Source: CAD feature listing. Evaluate the final solid. Frame: model axes, mm. Round coordinates to 2 decimals unless told otherwise and drop trailing zeros. Write each loop counter-clockwise with the first axis right and the second up, starting at its lowest first coordinate (ties: lowest second). Pieces come first, ordered by that corner, then holes. Notation, with made-up numbers: M 10.5,21.5 L 32.5,21.5 A20 cw 32.5,38.5 Z; hole C 13.25,-19.75 d1. An arc over 180 degrees is marked long. Answer in a Markdown table with one row per item. Add a question column.
Item 1: Cut plane B-B on x = 4.5. Return loops of the section in (y, z), and give its area (3 significant figures).
Item 2: Cut plane A-A on x = -20. Return loops of the section in (y, z).
Item 3: Contact query for flat-ended pins moving along their axis: pin 1 (1.5 mm diameter, centred on x = 76.5, z = 1, fed in from -Y); pin 2 (0.9 mm diameter, centred on x = -11, z = 1, fed in from +Y); pin 3 (0.9 mm diameter, centred on y = 53, z = 1, fed in from +X). Output: stop coordinate, or through.
Item 4: Cut plane C-C on y = -30. Return loops of the section in (x, z).
Item 5: Cut plane D-D on z = 0.6. Give the number of separate pieces and of enclosed holes in the cut face, and give its area (3 significant figures).
Item 6: Material intervals for probe 1 along Y at (x, z) = (-24, 1.3); probe 2 along Y at (x, z) = (-39, 0.15); probe 3 along X at (y, z) = (28, 2.7), sorted ascending.
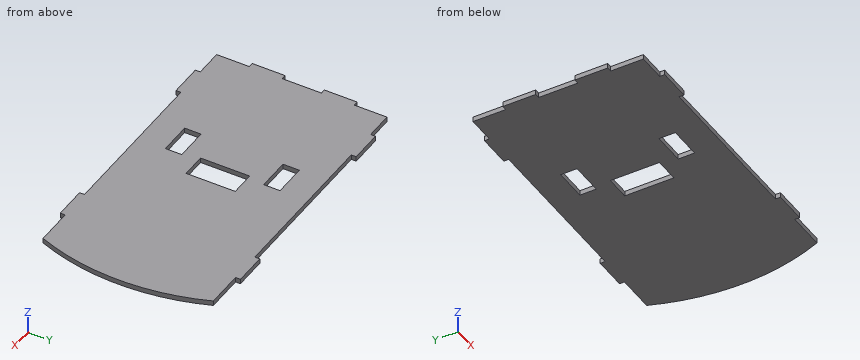
from build123d import *

# Parameters (mm, degrees)
SKETCH1_W           = 15
SKETCH1_H           = 30
SKETCH1_W_2         = 20
SKETCH1_H_2         = 10
BOSS_EXTRUDE1_DEPTH = 3


with BuildPart() as part:
    # Sketch1 → Boss-Extrude1 (new body)
    with BuildSketch(Plane.XY):
        with BuildLine():
            Line((-50, 52), (-50, 55))
            Line((-50, 55), (-70, 55))
            Line((-70, 55), (-70, 52))
            Line((-70, 52), (-87, 52))
            Line((-87, 52), (-87, 32))
            Line((-87, 32), (-90, 32))
            Line((-90, 32), (-90, 12))
            Line((-90, 12), (-87, 12))
            Line((-87, 12), (-87, -12))
            Line((-87, -12), (-90, -12))
            Line((-90, -12), (-90, -32))
            Line((-90, -32), (-87, -32))
            Line((-87, -32), (-87, -52))
            Line((-87, -52), (-70, -52))
            Line((-70, -52), (-70, -55))
            Line((-70, -55), (-50, -55))
            Line((-50, -55), (-50, -52))
            Line((-50, -52), (50, -52))
            Line((50, -52), (50, -55))
            Line((50, -55), (70, -55))
            Line((70, -55), (70, -52))
            Line((70, -52), (90, -52))
            Line((90, -52), (93, -52))
            ThreePointArc((93, -52), (103, 0), (93, 52))
            Line((93, 52), (90, 52))
            Line((90, 52), (70, 52))
            Line((70, 52), (70, 55))
            Line((70, 55), (50, 55))
            Line((50, 55), (50, 52))
            Line((50, 52), (-50, 52))
        make_face()
        Rectangle(SKETCH1_W, SKETCH1_H, mode=Mode.SUBTRACT)
        with Locations((-15, 30)):
            Rectangle(SKETCH1_W_2, SKETCH1_H_2, mode=Mode.SUBTRACT)
        with Locations((-15, -30)):
            Rectangle(SKETCH1_W_2, SKETCH1_H_2, mode=Mode.SUBTRACT)
    extrude(amount=BOSS_EXTRUDE1_DEPTH)


solid = part.part
Results below:
| question | item | result |
|---|---|---|
| 1 | outline | M -52,0 L -15,0 L -15,3 L -52,3 Z; M 15,0 L 52,0 L 52,3 L 15,3 Z |
| 1 | area | 222 mm2 |
| 2 | outline | M -52,0 L -35,0 L -35,3 L -52,3 Z; M -25,0 L 25,0 L 25,3 L -25,3 Z; M 35,0 L 52,0 L 52,3 L 35,3 Z |
| 3 | pin 1 | y = -52 |
| 3 | pin 2 | y = 52 |
| 3 | pin 3 | x = 70 |
| 4 | outline | M -90,0 L -25,0 L -25,3 L -90,3 Z; M -5,0 L 99.75,0 L 99.75,3 L -5,3 Z |
| 5 | separate pieces | 1 |
| 5 | enclosed holes | 3 |
| 5 | area | 18,900 mm2 |
| 6 | probe 1 | -52 to -35, -25 to 25, 35 to 52 |
| 6 | probe 2 | -52 to 52 |
| 6 | probe 3 | -90 to -25, -5 to 100.18 |
